Part model, mm, in its own coordinate system. Face numbers are marked on the shaded views. A direction names the side the tool comes from. Round coordinates to 2 decimals unless told otherwise and drop trailing zeros. Order: outer loops, then holes, each group sorted by start corner. A loop starts at its lowest first (then second) coordinate and runs counter-clockwise, first axis right, second up. Notation, with made-up numbers: M 32.25,-23 L 63.25,-23 A15 cw 63.25,6 Z; hole C 75,27.5 d11. An arc over 180 degrees is marked long. Write each question's results on one line, items separated by ' | '. Start each with the question number.
1. Probe L1, parallel to X at y = 0.25, z = -5; L2, parallel to Z at x = 1, y = 0 (3 decimals); L3, parallel to Y at x = 3, z = -35. List the from-to ranges inside material, lowest first. Write a range as [from, to].
2. Which spindle directions (+Z, -Z, +X, -X, +Y, -Y) get a long thin tool onto all of the face, cutting with end or side? Do the marked faces 1 and 2. Say none if no direction does.
3. Band-saw the part on A-A, the plane z = -42.5. List the corners of the cut face in (x, y), then the cut area to 3 significant figures.
4. Drop flat-ended pins along their axis: pin 1 Ø8 at (y, z) = (-9.5, -40) entering from +X; pin 2 Ø6 at (y, z) = (-4, -23.5) entering from +X; pin 3 Ø2 at (x, y) = (8.5, -3) entering from +Z; pin 4 Ø8 at (x, y) = (-7.5, -2.5) entering from -Z. Give the stop position or say it passes through.
```python
from build123d import *

# Parameters (mm, degrees)
F2_DEPTH = 12.7
F3_R     = 6.35
F4_DEPTH = 50.8


with BuildPart() as f1:
    # F0 (on Front) → F1 (revolve)
    with BuildSketch(Plane.XZ):
        with BuildLine():
            Line((0, 3.175), (0, 0))
            Line((0, 0), (12.7, 0))
            ThreePointArc((12.7, 0), (7.6159171285, 4.2838145072), (1.27, 6.2658087489))
            Line((1.27, 6.2658087489), (1.27, 3.175))
            Line((1.27, 3.175), (0, 3.175))
        make_face()
    revolve(axis=Axis((0, 0, 3.175), (0, 0, 1)))

    # F0 (on Front) → F2 (cut, symmetric)
    with BuildSketch(Plane.XZ):
        with BuildLine():
            Line((-1.27, 3.175), (0, 3.175))
            Line((0, 3.175), (0, 6.35))
            ThreePointArc((0, 6.35), (0.6357958012, 6.3199087984), (1.27, 6.2658087489))
            Line((1.27, 6.2658087489), (1.27, 9.525))
            Line((1.27, 9.525), (-1.27, 9.525))
            Line((-1.27, 9.525), (-1.27, 3.175))
        make_face()
        with BuildLine():
            Line((0, 6.35), (0, 3.175))
            Line((0, 3.175), (1.27, 3.175))
            Line((1.27, 3.175), (1.27, 6.2658087489))
            ThreePointArc((1.27, 6.2658087489), (0.6357958012, 6.3199087984), (0, 6.35))
        make_face()
    extrude(amount=F2_DEPTH, both=True, mode=Mode.SUBTRACT)

    # F3 (on face) → F4 (join)
    with BuildSketch(Plane(origin=(0, 0, 0), x_dir=(1, 0, 0), z_dir=(0, 0, -1))):
        Circle(F3_R)
    extrude(amount=F4_DEPTH)


solid = f1.part
```
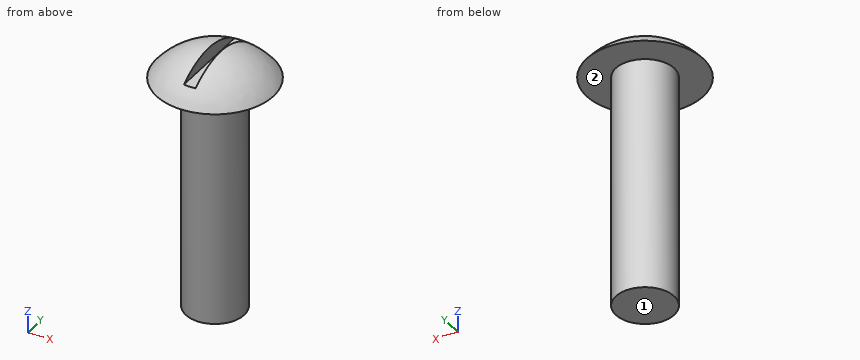
Solution:
1) L1: [-6.35, 6.35] | L2: [-50.8, 3.175] | L3: [-5.6, 5.6]
2) face 1: -Z, +X, -X, +Y, -Y | face 2: -Z
3) outline: C 0,0 d12.7 | area: 127 mm^2
4) pin 1: x = 3.17 | pin 2: x = 6.27 | pin 3: z = 4.06 | pin 4: z = -50.8
